For this review, take the finished solid that the model builds, in its own axes (mm). Round coordinates to 2 decimals unless told otherwise and drop trailing zeros. Order: outer loops, then holes, each group sorted by start corner. A loop starts at its lowest first (then second) coordinate and runs counter-clockwise, first axis right, second up. Notation, with made-up numbers: M 89,-25 L 115,-25 A19 ccw 115,-8 Z; hole C 62,71 d7. An arc over 180 degrees is marked long. Answer as a JSON object with one key per item and string values.
from build123d import *

# Parameters (mm, degrees)
SKETCH1_W           = 177.8
SKETCH1_H           = 101.6
BOSS_EXTRUDE1_DEPTH = 6.35
SKETCH2_R           = 1.5875
CUT_EXTRUDE1_DEPTH  = 6.35
SKETCH5_R           = 5.499261314
CUT_EXTRUDE3_DEPTH  = 6.35


with BuildPart() as part:
    # Sketch1 → Boss-Extrude1 (new body)
    with BuildSketch(Plane.XY):
        with Locations((88.9, 50.8)):
            Rectangle(SKETCH1_W, SKETCH1_H)
    extrude(amount=BOSS_EXTRUDE1_DEPTH)

    # Sketch2 → Cut-Extrude1 (cut)
    with BuildSketch(Plane.XY.offset(6.35)):
        with Locations((6.35, 81.28)):
            Circle(SKETCH2_R)
        with Locations((6.35, 60.96)):
            Circle(SKETCH2_R)
        with Locations((6.35, 40.64)):
            Circle(SKETCH2_R)
        with Locations((6.35, 20.32)):
            Circle(SKETCH2_R)
        with Locations((171.45, 20.32)):
            Circle(SKETCH2_R)
        with Locations((171.45, 40.64)):
            Circle(SKETCH2_R)
        with Locations((171.45, 60.96)):
            Circle(SKETCH2_R)
        with Locations((171.45, 81.28)):
            Circle(SKETCH2_R)
    extrude(amount=-CUT_EXTRUDE1_DEPTH, mode=Mode.SUBTRACT)

    # Sketch5 → Cut-Extrude3 (cut)
    with BuildSketch(Plane.XY.offset(6.35)):
        with Locations((120.65, 50.8)):
            Circle(SKETCH5_R)
        with Locations((57.15, 50.8)):
            Circle(SKETCH5_R)
    extrude(amount=-CUT_EXTRUDE3_DEPTH, mode=Mode.SUBTRACT)


solid = part.part
1) Add section A-A on x = 57.15. State the section outline as (y, z) points.
Geometry check:
{"outline": "M 0,0 L 45.3,0 L 45.3,6.35 L 0,6.35 Z; M 56.3,0 L 101.6,0 L 101.6,6.35 L 56.3,6.35 Z"}
2) Add section C-C on x = 118.5. State the section outline as (y, z) points, and give its area (3 significant figures).
Geometry check:
{"outline": "M 0,0 L 45.74,0 L 45.74,6.35 L 0,6.35 Z; M 55.86,0 L 101.6,0 L 101.6,6.35 L 55.86,6.35 Z", "area": "581 mm²"}
3) For L1, parallel to X at y = 81.28, z = 1.75; L2, parallel to Y at x = 6.35, z = 3.75; L3, parallel to X at y = 48.5, z = 3, list the stretches that pass through material, from the lowest coordinate up.
Geometry check:
{"L1": "x = 0 to 4.76, 7.94 to 169.86, 173.04 to 177.8", "L2": "y = 0 to 18.73, 21.91 to 39.05, 42.23 to 59.37, 62.55 to 79.69, 82.87 to 101.6", "L3": "x = 0 to 52.15, 62.15 to 115.65, 125.65 to 177.8"}
4) Add section B-B on y = 50.8. State the section outline as (x, z) points, and give its area (3 significant figures).
Geometry check:
{"outline": "M 0,0 L 51.65,0 L 51.65,6.35 L 0,6.35 Z; M 62.65,0 L 115.15,0 L 115.15,6.35 L 62.65,6.35 Z; M 126.15,0 L 177.8,0 L 177.8,6.35 L 126.15,6.35 Z", "area": "989 mm²"}
5) Mouldability with a two-part tool opening along Y and no side actions: class faces 1 (the cylindrical face through (119.46, 45.43, 3.22)), 2 (the flat face through (88, 101.6, 3)), 3 (the flat face through (88, 52, 6.35)) as +Y half, -Y half, draft (parallel to the pull), parting line (faces both ways), or undercut.
Geometry check:
{"face 1": "undercut", "face 2": "+Y half", "face 3": "draft"}
